```python
from build123d import *

# Parameters (mm, degrees)
SKETCH1_R           = 12
SKETCH1_R_2         = 1.55
SKETCH1_R_3         = 3.65
SKETCH1_R_4         = 2.55
SKETCH1_R_5         = 2.05
BOSS_EXTRUDE1_DEPTH = 6.3
FILLET1_R           = 5


with BuildPart() as part:
    # Sketch1 → Boss-Extrude1 (new body)
    with BuildSketch(Plane(origin=(0, 0, 0), x_dir=(1, 0, 0), z_dir=(0, 1, 0))):
        Polygon((0, 0), (99, 0), (99, 81.5), (79, 81.5), (79, 128.5), (37, 128.5), (37, 81.5), (0, 81.5), align=None)
        with Locations(Location((58, 107.5, 0), (0, 0, 270))):
            Circle(SKETCH1_R, mode=Mode.SUBTRACT)
        with Locations(Location((42.5, 123, 0), (0, 0, 270))):
            Circle(SKETCH1_R_2, mode=Mode.SUBTRACT)
        with Locations(Location((73.5, 123, 0), (0, 0, 270))):
            Circle(SKETCH1_R_2, mode=Mode.SUBTRACT)
        with Locations(Location((73.5, 92, 0), (0, 0, 270))):
            Circle(SKETCH1_R_2, mode=Mode.SUBTRACT)
        with Locations(Location((42.5, 92, 0), (0, 0, 270))):
            Circle(SKETCH1_R_2, mode=Mode.SUBTRACT)
        with Locations(Location((10, 71.5, 0), (0, 0, 270))):
            Circle(SKETCH1_R_3, mode=Mode.SUBTRACT)
        with Locations(Location((89, 71.5, 0), (0, 0, 270))):
            Circle(SKETCH1_R_3, mode=Mode.SUBTRACT)
        with Locations(Location((89, 10, 0), (0, 0, 270))):
            Circle(SKETCH1_R_4, mode=Mode.SUBTRACT)
        with Locations(Location((10, 10, 0), (0, 0, 270))):
            Circle(SKETCH1_R_4, mode=Mode.SUBTRACT)
        with Locations(Location((40, 66.5, 0), (0, 0, 270))):
            Circle(SKETCH1_R_5, mode=Mode.SUBTRACT)
        with Locations(Location((60, 66.5, 0), (0, 0, 270))):
            Circle(SKETCH1_R_5, mode=Mode.SUBTRACT)
        with Locations(Location((60, 15, 0), (0, 0, 270))):
            Circle(SKETCH1_R_5, mode=Mode.SUBTRACT)
        with Locations(Location((40, 15, 0), (0, 0, 270))):
            Circle(SKETCH1_R_5, mode=Mode.SUBTRACT)
    extrude(amount=BOSS_EXTRUDE1_DEPTH)

    # Fillet1
    fillet1_edges = [part.edges().sort_by_distance(p)[0] for p in [
        (0, 3.15, -81.5),
        (37, 3.15, -81.5),
        (37, 3.15, -128.5),
        (79, 3.15, -128.5),
        (79, 3.15, -81.5),
        (99, 3.15, -81.5),
        (99, 3.15, 0),
        (0, 3.15, 0),
    ]]
    fillet(fillet1_edges, radius=FILLET1_R)


solid = part.part
```
Check sheet for the modelled part. Datum: model origin and axes. Units: mm. A direction names the side the tool comes from. Coordinates: 2 decimals unless noted, no trailing zeros. Write each loop counter-clockwise with the first axis right and the second up, starting at its lowest first coordinate (ties: lowest second). Pieces come first, ordered by that corner, then holes. Notation, with made-up numbers: (63.5, 12.5) -> (92.5, 12.5) arc R18 ccw to (92.5, 41.5) -> close; hole circle Ø10 at (11.25, -39). An arc over 180 degrees is marked (long way). Use a Markdown table: item, result.
1. Sectioned sample at D-D (z = -115.5). Enter the section's corners in (x, y), plus the area to 3 significant figures.
Reported:
| item | result |
|---|---|
| outline | (37, 0) -> (49.06, 0) -> (49.06, 6.3) -> (37, 6.3) -> close; (66.94, 0) -> (79, 0) -> (79, 6.3) -> (66.94, 6.3) -> close |
| area | 152 mm2 |
2. Sectioned sample at B-B (z = -10). Enter the section's corners in (x, y), plus the area to 3 significant figures.
Reported:
| item | result |
|---|---|
| outline | (0, 0) -> (7.45, 0) -> (7.45, 6.3) -> (0, 6.3) -> close; (12.55, 0) -> (86.45, 0) -> (86.45, 6.3) -> (12.55, 6.3) -> close; (91.55, 0) -> (99, 0) -> (99, 6.3) -> (91.55, 6.3) -> close |
| area | 559 mm2 |
3. Release check for a two-part mould opening along X. For faces 1 (the flat face through (49, 0, -51)), 2 (the cylindrical face through (7.51, 3.11, -10.55)), 3 (the cylindrical face through (2, 3, -1)) record: pulls with the +X half, pulls with the -X half, needs draft (parallel to the pull), parting line crosses it, or undercut.
Reported:
| item | result |
|---|---|
| face 1 | needs draft |
| face 2 | undercut |
| face 3 | pulls with the -X half |
4. Tool access check on faces 4 (the cylindrical face through (92.08, 3.11, -69.54)), 5 (the flat face through (79, 3, -105)). Record the directions out of +Z, -Z, +X, -X, +Y, -Y that give a thin tool (end or side, any length) a straight path to the whole face; none if there is none.
Reported:
| item | result |
|---|---|
| face 4 | +Y, -Y |
| face 5 | -Z, +X, +Y, -Y |
5. Go/stop test with flat-tipped pins: pin 1 Ø3 at (y, z) = (3.5, -98) entering from -X; pin 2 Ø3 at (x, y) = (13, 2) entering from -Z. Record where each tip stops, or that it passes through.
Reported:
| item | result |
|---|---|
| pin 1 | stops at x = 37 |
| pin 2 | stops at z = -81.5 |
6. Sectioned sample at C-C (y = 4.5). Give the number of separate pieces and of enclosed holes in the cut face, plus the area to 3 significant figures.
Reported:
| item | result |
|---|---|
| separate pieces | 1 |
| enclosed holes | 13 |
| area | 9,360 mm2 |
7. Sectioned sample at A-A (x = 10). Enter the section's corners in (y, z), plus the area to 3 significant figures.
Reported:
| item | result |
|---|---|
| outline | (0, -81.5) -> (6.3, -81.5) -> (6.3, -75.15) -> (0, -75.15) -> close; (0, -67.85) -> (6.3, -67.85) -> (6.3, -12.55) -> (0, -12.55) -> close; (0, -7.45) -> (6.3, -7.45) -> (6.3, 0) -> (0, 0) -> close |
| area | 435 mm2 |
8. Scan lines: line 1 along X through (y, z) = (5.25, -10); line 2 along X through (y, z) = (3.5, -123); line 3 along Z through (x, y) = (9, 2.5). Record each from-to range of solid material in increasing order.
Reported:
| item | result |
|---|---|
| line 1 | x = 0 to 7.45, 12.55 to 86.45, 91.55 to 99 |
| line 2 | x = 37 to 40.95, 44.05 to 71.95, 75.05 to 79 |
| line 3 | z = -81.5 to -75.01, -67.99 to -12.35, -7.65 to 0 |
